Autodesk Inventor part; units mm, degrees
ref_plane "YZ Plane" through (0, 0, 0) normal (1, 0, 0) x (0, 1, 0)
ref_plane "XZ Plane" through (0, 0, 0) normal (0, 1, 0) x (-1, 0, 0)
ref_plane "XY Plane" through (0, 0, 0) normal (0, 0, 1) x (1, 0, 0)
sketch "Sketch1" plane through (0, 0, 0) normal (0, 0, 1) x (1, 0, 0)
  circle A0 centre (0, 0) radius 60
  dimension "d0" = 120
extrude "Extrusion1" add sketch "Sketch1" along normal blind 5.8
sketch "Sketch2" plane through (0, 0, 5.8) normal (0, 0, 1) x (1, 0, 0)
  circle A0 centre (0, 0) radius 60
  circle A1 centre (0, 0) radius 6.4031
extrude "Extrusion2" cut sketch "Sketch2" against normal through all contours A1
sketch "Sketch3" plane through (0, 0, 0) normal (0, 0, -1) x (-1, 0, 0)
  circle A0 centre (0, 0) radius 6.4031
  circle A1 centre (0, 0) radius 3
  line L0 (12.25, 9.9) -> (-28.05, 9.9)
  line L1 (-28.05, -9.9) -> (12.25, -9.9)
  line L2 (-28.05, 9.9) -> (-28.05, -9.9)
  line L3 (18.25, 2.5) -> (12.25, 2.5)
  line L4 (18.25, -2.5) -> (18.25, 2.5)
  line L5 (12.25, -2.5) -> (18.25, -2.5)
  line L6 (12.25, 2.5) -> (12.25, 9.9)
  line L7 (12.25, -9.9) -> (12.25, -2.5)
extrude "Extrusion3" cut sketch "Sketch3" against normal through all contours L6 L3 L4 L5 L7 L1 L2 L0
sketch "Sketch4" plane through (0, 0, 5.8) normal (0, 0, 1) x (1, 0, 0)
  circle A0 centre (-16.6, 5) radius 2.5
  circle A1 centre (-16.6, -5) radius 2.5
  circle A2 centre (32.4, -5) radius 2.5
  circle A3 centre (32.4, 5) radius 2.5
  circle A4 centre (-16.6, 5) radius 1.5
  circle A5 centre (-16.6, -5) radius 1.5
  circle A6 centre (32.4, 5) radius 1.5
  circle A7 centre (32.4, -5) radius 1.5
  dimension "d7" = 3
  dimension "d8" = 3
  dimension "d9" = 3
  dimension "d10" = 3
extrude "Extrusion4" cut sketch "Sketch4" against normal through all contours A4 | A5 | A6 | A7
sketch "Sketch5" plane through (0, 0, 5.8) normal (0, 0, 1) x (1, 0, 0)
  circle A0 centre (0, 0) radius 60
  circle A1 centre (-35.355, 35.355) radius 1.5
  line L0 (0, -84) -> (0, 84)
  line L1 (-84, 0) -> (84, 0)
  circle A2 centre (-35.355, -35.355) radius 1.5
  circle A3 centre (35.355, -35.355) radius 1.5
  circle A4 centre (35.355, 35.355) radius 1.5
  dimension "d13" = 3
  dimension "d15" = 35.355
  dimension "d17" = 35.355
  dimension "d20" = 360
extrude "Extrusion5" cut sketch "Sketch5" against normal through all contours A1 | A2 | A3 | A4
sketch "Sketch6" plane through (0, 0, 0) normal (0, 0, -1) x (-1, 0, 0)
  circle A0 centre (-35.355, 35.355) radius 1.5
  circle A1 centre (-35.355, -35.355) radius 1.5
  circle A2 centre (35.355, -35.355) radius 1.5
  circle A3 centre (35.355, 35.355) radius 1.5
  circle A4 centre (-32.4, 5) radius 1.5
  circle A5 centre (16.6, -5) radius 1.5
  circle A6 centre (16.6, 5) radius 1.5
  circle A7 centre (-32.4, -5) radius 1.5
  line L0 (-28.05, -9.9) -> (-28.05, 9.9)
  line L1 (-28.05, 9.9) -> (12.25, 9.9)
  line L2 (12.25, 9.9) -> (12.25, 2.5)
  line L3 (12.25, 2.5) -> (18.25, 2.5)
  line L4 (18.25, 2.5) -> (18.25, -2.5)
  line L5 (18.25, -2.5) -> (12.25, -2.5)
  line L6 (12.25, -2.5) -> (12.25, -9.9)
  line L7 (12.25, -9.9) -> (-28.05, -9.9)
  circle A8 centre (0, 0) radius 60
  circle A9 centre (35.355, 35.355) radius 1.385
  circle A10 centre (-35.355, 35.355) radius 1.5
  circle A11 centre (-35.355, -35.355) radius 1.5
  circle A12 centre (35.355, -35.355) radius 1.5
  circle A13 centre (35.355, 35.355) radius 1.5
  circle A14 centre (-32.4, 5) radius 1.5
  circle A15 centre (16.6, -5) radius 1.5
  circle A16 centre (16.6, 5) radius 1.5
  circle A17 centre (-32.4, -5) radius 1.5
  line L8 (-28.05, -9.9) -> (-28.05, 9.9)
  line L9 (-28.05, 9.9) -> (12.25, 9.9)
  line L10 (12.25, 9.9) -> (12.25, 2.5)
  line L11 (12.25, 2.5) -> (18.25, 2.5)
  line L12 (18.25, 2.5) -> (18.25, -2.5)
  line L13 (18.25, -2.5) -> (12.25, -2.5)
  line L14 (12.25, -2.5) -> (12.25, -9.9)
  line L15 (12.25, -9.9) -> (-28.05, -9.9)
  circle A18 centre (0, 0) radius 60
  line L16 (-28.05, 9.9) -> (-28.05, -9.9)
  line L17 (-28.05, -9.9) -> (-28.05, 9.9)
  line L18 (12.25, 9.9) -> (-28.05, 9.9)
  line L19 (-28.05, 9.9) -> (12.25, 9.9)
  circle A19 centre (-32.4, -5) radius 1.5
  circle A20 centre (-32.4, -5) radius 1.5
  circle A21 centre (35.355, -35.355) radius 1.385
  circle A22 centre (-35.355, 35.355) radius 1.385
  circle A23 centre (-35.355, -35.355) radius 1.385
equation "\"d17\" = d15"
properties part number "Acrylic_rotationServoMount"
Could you check a few things on this model? Use its own coordinates, in mm. A direction names the side the tool comes from. Give positions to 0.01 mm unless a question says otherwise; leave off trailing zeros. Order: outer loops, then holes, each group sorted by start corner. A loop starts at its lowest first (then second) coordinate and runs counter-clockwise, first axis right, second up.
1. Suppose I cut it at C-C (z = 4.6). Give the number of separate pieces and of enclosed holes in the cut face, plus the area to 3 significant figures.
2. For faces 4 (the flat face through (8, -9.9, 3)), 5 (the flat face through (-1, -12, 0)), which set-ups out of +Z, -Z, +X, -X, +Y, -Y let a thin tool reach every point of the face, with its end or its side?
3. I need wall thicknesses on L1, parallel to Y at x = 0.5, z = 3.35; L2, parallel to Y at x = -16.6, z = 3.2; L3, parallel to Y at x = 32.4, z = 4.2. Which ranges of each line are inside material? Lowest first, please.
4. Suppose I cut it at B-B (y = 0). List the corners of the cut face in (x, z) for me, plus the area to 3 significant figures.
5. Will these pins go through, and if not, where does the flat tip stop? P1, Ø1.7, axis at x = -14, z = 1.5, coming from the -Y side; P2, Ø1.5, axis at y = -31, z = 0.5, coming from the -X side; P3, Ø1.7, axis at y = 4.5, z = 4, coming from the -X side.
6. We'd pull the mould along X, two halves only. Please class faces 1 (the flat face through (-1, -12, 5.8)), 2 (the cylindrical face through (33.83, -4.55, 2.94)), 3 (the cylindrical face through (-59.94, -2.64, 2.86)): pulls with the +X half, pulls with the -X half, needs draft (parallel to the pull), parting line crosses it, or undercut.
7. Suppose I cut it at D-D (x = 32.4). List the corners of the cut face in (y, z) for me, plus the area to 3 significant figures.
8. Suppose I cut it at A-A (x = 0). List the corners of the cut face in (y, z) for me, plus the area to 3 significant figures.
Solved:
1. separate pieces: 1
1. enclosed holes: 9
1. area: 10,400 mm2
2. face 4: +Z, -Z
2. face 5: -Z, +X, -X, +Y, -Y
3. L1: y = -60 to -9.9, 9.9 to 60
3. L2: y = -57.66 to -6.5, -3.5 to -2.5, 2.5 to 3.5, 6.5 to 57.66
3. L3: y = -50.5 to -6.5, -3.5 to 3.5, 6.5 to 50.5
4. outline: (-60, 0) - (-18.25, 0) - (-18.25, 5.8) - (-60, 5.8) - close; (28.05, 0) - (60, 0) - (60, 5.8) - (28.05, 5.8) - close
4. area: 427 mm2
5. P1: stops at y = -58.54
5. P2: stops at x = -51.82
5. P3: stops at x = -59.89
6. face 1: needs draft
6. face 2: undercut
6. face 3: parting line crosses it
7. outline: (-50.5, 0) - (-6.5, 0) - (-6.5, 5.8) - (-50.5, 5.8) - close; (-3.5, 0) - (3.5, 0) - (3.5, 5.8) - (-3.5, 5.8) - close; (6.5, 0) - (50.5, 0) - (50.5, 5.8) - (6.5, 5.8) - close
7. area: 551 mm2
8. outline: (-60, 0) - (-9.9, 0) - (-9.9, 5.8) - (-60, 5.8) - close; (9.9, 0) - (60, 0) - (60, 5.8) - (9.9, 5.8) - close
8. area: 581 mm2
